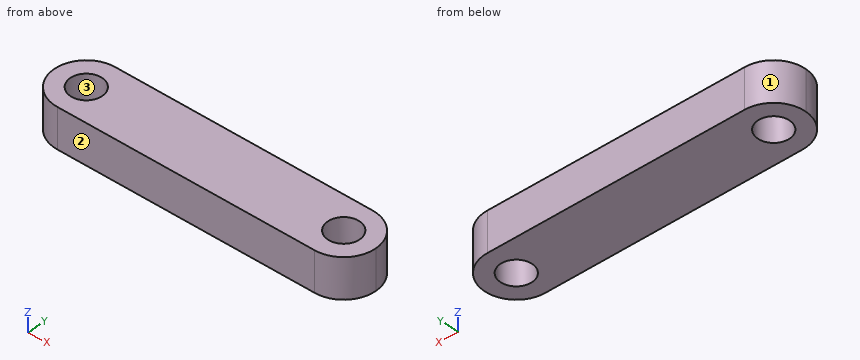
```python
from build123d import *

# Parameters (mm, degrees)
F0_W     = 127
F0_H     = 25.4
F1_DEPTH = 15.875
F2_R     = 6.35
F3_DEPTH = 15.876
F4_R     = 12.69999
F5_R     = 6.35
F6_DEPTH = 15.876
F7_R     = 12.69999


# Not quite as in the source:
# - a fillet or chamfer is up to 0.001 mm smaller than in the source, because OpenCascade refuses the exact size


with BuildPart() as f1:
    # F0 (on Top) → F1 (new body)
    with BuildSketch(Plane.XY):
        with Locations((65.2798527717, 12.1217946971)):
            Rectangle(F0_W, F0_H)
    extrude(amount=F1_DEPTH)

    # F2 (on face) → F3 (cut, through all)
    with BuildSketch(Plane(origin=(0, 0, 0), x_dir=(1, 0, 0), z_dir=(0, 0, -1))):
        with Locations((116.0798527717, -12.1217946971)):
            Circle(F2_R)
    extrude(amount=-F3_DEPTH, mode=Mode.SUBTRACT)

    # F4 (radius 12.7 in the source; OpenCascade refuses exactly that, so slightly less here)
    f4_edges = [f1.edges().sort_by_distance(p)[0] for p in [
        (128.779853, 24.821795, 7.9375),
        (128.779853, -0.578205, 7.9375),
    ]]
    fillet(f4_edges, radius=F4_R)

    # F5 (on face) → F6 (cut, through all)
    with BuildSketch(Plane.XY.offset(15.875)):
        with Locations((14.4798527717, 12.1217946971)):
            Circle(F5_R)
    extrude(amount=-F6_DEPTH, mode=Mode.SUBTRACT)

    # F7 (radius 12.7 in the source; OpenCascade refuses exactly that, so slightly less here)
    f7_edges = [f1.edges().sort_by_distance(p)[0] for p in [
        (1.779853, 24.821795, 7.9375),
        (1.779853, -0.578205, 7.9375),
    ]]
    fillet(f7_edges, radius=F7_R)


solid = f1.part
```
Source: CAD feature listing. Evaluate the final solid. Frame: model axes, mm. Face numbers are marked on the shaded views. Give positions to 0.01 mm unless a question says otherwise; leave off trailing zeros. Loops run counter-clockwise (first coordinate to the right, second up) from the corner with the lowest first, then second, coordinate; pieces in that order, holes last. Notation, with made-up numbers: (-3, 34.5) - (39, 34.5) arc R25 cw to (39, 50.5) - close; hole circle Ø10 at (-30, -22). An arc over 180 degrees is marked (long way). Use CSV: the item, a comma, the result in double quotes.
1) Pin query (flat end, axial travel): P1, Ø10, axis at x = 116.08, y = 12.12, coming from the +Z side; P2, Ø1.5, axis at y = 16.5, z = 14, coming from the -X side; P3, Ø6, axis at y = 3, z = 8.5, coming from the +X side; P4, Ø5, axis at y = 4.5, z = 12.5, coming from the +X side. Return the tip coordinate at first contact, or that it passes through.
Worked out:
P1,"passes through"
P2,"stops at x = 2.31"
P3,"stops at x = 127.21"
P4,"stops at x = 127.7"
2) Line query: line 1 (X direction, y = 11.5, z = 8.5); line 2 (X direction, y = 11.25, z = 3.5); line 3 (Y direction, x = 11.5, z = 8). Output: solid intervals per line, ascending.
Worked out:
line 1,"x = 1.8 to 8.16, 20.8 to 109.76, 122.4 to 128.76"
line 2,"x = 1.81 to 8.19, 20.77 to 109.79, 122.37 to 128.75"
line 3,"y = -0.22 to 6.51, 17.73 to 24.47"
3) Mould query, pull axis X, two halves, no side actions, for the marked faces 1, 2 and 3. Classes: +X half, -X half, draft (parallel to the pull), parting line (faces both ways), or undercut.
Worked out:
face 1,"-X half"
face 2,"draft"
face 3,"undercut"
4) Cut plane B-B (y = 8.25). Output: boundary loops of the cut face in (x, z) (3 decimals), and give its area (3 significant figures).
Worked out:
outline,"(2.384, 0) - (9.447, 0) - (9.447, 15.875) - (2.384, 15.875) - close; (19.513, 0) - (111.047, 0) - (111.047, 15.875) - (19.513, 15.875) - close; (121.113, 0) - (128.175, 0) - (128.175, 15.875) - (121.113, 15.875) - close"
area,"1,680 mm^2"
5) Cut plane C-C (y = 13.5). Output: boundary loops of the cut face in (x, z) (3 decimals).
Worked out:
outline,"(1.855, 0) - (8.281, 0) - (8.281, 15.875) - (1.855, 15.875) - close; (20.678, 0) - (109.881, 0) - (109.881, 15.875) - (20.678, 15.875) - close; (122.278, 0) - (128.705, 0) - (128.705, 15.875) - (122.278, 15.875) - close"
6) Cut plane A-A (z = 6.25). Count the separate pieces of the cut face and the enclosed holes in it, and give its area (3 significant figures).
Worked out:
separate pieces,"1"
enclosed holes,"2"
area,"2,830 mm^2"
7) Cut plane D-D (y = 3.5). Output: boundary loops of the cut face in (x, z) (3 decimals), and give its area (3 significant figures).
Worked out:
outline,"(5.155, 0) - (125.405, 0) - (125.405, 15.875) - (5.155, 15.875) - close"
area,"1,910 mm^2"
